Here's how the part is built. I have some questions about the finished solid (model axes, mm). Face numbers are marked on the shaded views. A direction names the side the tool comes from. Coordinates: 2 decimals unless noted, no trailing zeros. Loops run counter-clockwise (first coordinate to the right, second up) from the corner with the lowest first, then second, coordinate; pieces in that order, holes last. Notation, with made-up numbers: M 10.25,88 L 18.25,88 A10 ccw 18.25,92 Z; hole C 81,58 d5. An arc over 180 degrees is marked long. Use CSV: the item, a comma, the result in double quotes. Start each with the question number.
Q1. Which directions (+Z, -Z, +X, -X, +Y, -Y) give clear straight access to the entire face, cutting with the end or side of a thin tool? Please do the marked faces 4, 5, 6 and 7.
Q2. If we section it at B-B (z = 1.8): Please give me the cut outline in (x, y).
Q3. If we section it at A-A (z = 2.4): Please give me the cut outline in (x, y), and give its area (3 significant figures).
Q4. Please list where these lines run through material, in increasing order: probe 1 along Y at (x, z) = (0, 1.2); probe 2 along Y at (x, z) = (-2.5, 2.5); probe 3 along X at (y, z) = (0.25, 0.7). Write a range as [from, to].
Q5. For pin 1 Ø0.6 at (x, z) = (0, 1) entering from +Y; pin 2 Ø1 at (y, z) = (4.5, 1) entering from +X; pin 3 Ø1 at (y, z) = (-5.5, 2) entering from +X, each with a flat end and sliding along its axis, tell me the tip position at first contact or that it passes through.
Q6. If we mould it in two halves opening along Y, with no side actions, what happens to the marked faces 1, 2 and 3? For each: +Y half, -Y half, draft (parallel to the pull), parting line (faces both ways), or undercut.
from build123d import *

# Parameters (mm, degrees)
F0_R     = 3
F1_DEPTH = 3
F2_SIZE  = 0.99999


# Not quite as in the source:
# - a fillet or chamfer is up to 0.001 mm smaller than in the source, because OpenCascade refuses the exact size


with BuildPart() as f1:
    # F0 (on Top) → F1 (new body)
    with BuildSketch(Plane.XY):
        with BuildLine():
            Line((-1, 5), (-1, 5.9160797831))
            ThreePointArc((-1, 5.9160797831), (-4.2426406871, 4.2426406871), (-5.9160797831, 1))
            Line((-5.9160797831, 1), (-5, 1))
            Line((-5, 1), (-5, -1))
            Line((-5, -1), (-5.9160797831, -1))
            ThreePointArc((-5.9160797831, -1), (-4.2426406871, -4.2426406871), (-1, -5.9160797831))
            Line((-1, -5.9160797831), (-1, -5))
            Line((-1, -5), (1, -5))
            Line((1, -5), (1, -5.9160797831))
            ThreePointArc((1, -5.9160797831), (4.2426406871, -4.2426406871), (5.9160797831, -1))
            Line((5.9160797831, -1), (5, -1))
            Line((5, -1), (5, 1))
            Line((5, 1), (5.9160797831, 1))
            ThreePointArc((5.9160797831, 1), (4.2426406871, 4.2426406871), (1, 5.9160797831))
            Line((1, 5.9160797831), (1, 5))
            Line((1, 5), (-1, 5))
        make_face()
        Circle(F0_R, mode=Mode.SUBTRACT)
    extrude(amount=F1_DEPTH)

    # F2 (size 1 in the source; OpenCascade refuses exactly that, so slightly less here)
    f2_edges = [f1.edges().sort_by_distance(p)[0] for p in [
        (-4.242641, -4.242641, 3),
        (-4.242641, 4.242641, 3),
        (4.242641, 4.242641, 3),
        (4.242641, -4.242641, 3),
    ]]
    chamfer(f2_edges, length=F2_SIZE)


solid = f1.part
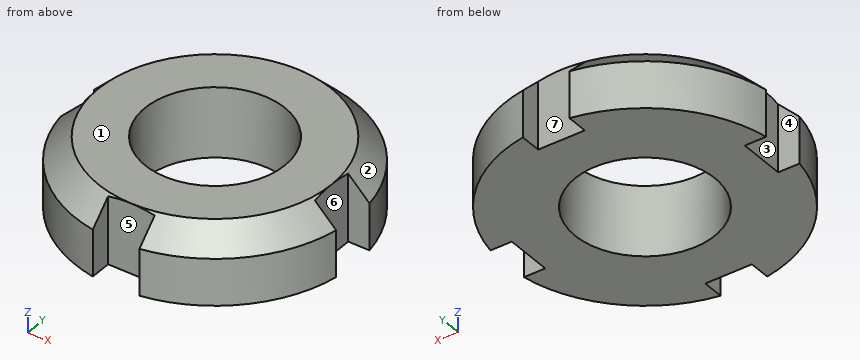
Results below:
1,face 4,"+Z, -Z, -X"
1,face 5,"+Z, -Z, -Y"
1,face 6,"+Z, -Z, +X"
1,face 7,"+Z, -Z, +Y"
2,outline,"M -5.92,-1 A6 ccw -1,-5.92 L -1,-5 L 1,-5 L 1,-5.92 A6 ccw 5.92,-1 L 5,-1 L 5,1 L 5.92,1 A6 ccw 1,5.92 L 1,5 L -1,5 L -1,5.92 A6 ccw -5.92,1 L -5,1 L -5,-1 Z; hole C 0,0 d6"
3,outline,"M -5.51,-1 A5.6 ccw -1,-5.51 L -1,-5 L 1,-5 L 1,-5.51 A5.6 ccw 5.51,-1 L 5,-1 L 5,1 L 5.51,1 A5.6 ccw 1,5.51 L 1,5 L -1,5 L -1,5.51 A5.6 ccw -5.51,1 L -5,1 L -5,-1 Z; hole C 0,0 d6"
3,area,"65.7 mm^2"
4,probe 1,"[-5, -3], [3, 5]"
4,probe 2,"[-4.9, -1.66], [1.66, 4.9]"
4,probe 3,"[-5, -2.99], [2.99, 5]"
5,pin 1,"y = 5"
5,pin 2,"x = 4.47"
5,pin 3,"x = 3.32"
6,face 1,"draft"
6,face 2,"+Y half"
6,face 3,"undercut"
